Input: dimensioned drawing with shaded views. Units: mm. Origin: part minimum x, y, z. A direction names the side the tool comes from. Coordinates: 2 decimals unless noted, no trailing zeros. Order: outer loops, then holes, each group sorted by start corner. A loop starts at its lowest first (then second) coordinate and runs counter-clockwise, first axis right, second up. Notation, with made-up numbers: (69, 75) -> (124, 75) arc R19 cw to (124, 101) -> close; hole circle Ø10 at (60, 0). An arc over 180 degrees is marked (long way). Answer as CSV lines item,"result".
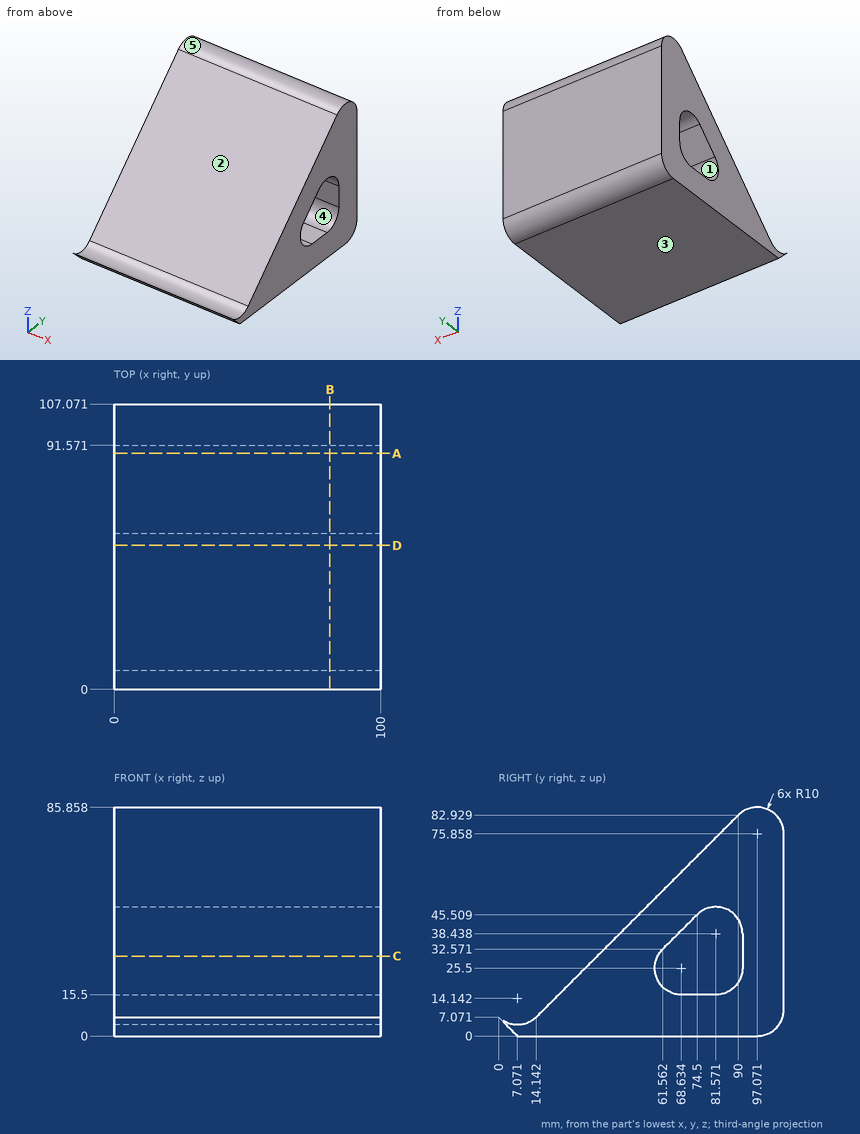
1. Contact query for flat-ended pins moving along their axis: pin 1 (14 mm diameter, centred on x = 53.5, y = 78, fed in from +Z); pin 2 (6.5 mm diameter, centred on x = 44.5, z = 29.5, fed in from -Y); pin 3 (12 mm diameter, centred on x = 54, y = 13.5, fed in from +Z). Output: stop coordinate, or through.
Findings:
pin 1,"stops at z = 77.93"
pin 2,"stops at y = 33.32"
pin 3,"stops at z = 12.43"
2. Cut plane D-D (y = 54). Return the cut outline in (x, z).
Findings:
outline,"(0, 0) -> (100, 0) -> (100, 46.93) -> (0, 46.93) -> close"
3. Mould query, pull axis Z, two halves, no side actions, for the marked faces 1, 2 and 3. Classes: released by +Z, released by -Z, zero draft, split by the parting line, or undercut.
Findings:
face 1,"undercut"
face 2,"released by +Z"
face 3,"released by -Z"
4. Cut plane C-C (z = 30). Return the cut outline in (x, y), plus the area to 3 significant figures.
Findings:
outline,"(0, 37.07) -> (100, 37.07) -> (100, 59.7) -> (0, 59.7) -> close; (0, 91.57) -> (100, 91.57) -> (100, 107.07) -> (0, 107.07) -> close"
area,"3,810 mm2"
5. Cut plane B-B (x = 81). Return the cut outline in (y, z), plus the area to 3 significant figures.
Findings:
outline,"(0, 7.07) -> (7.07, 0) -> (97.07, 0) arc R10 ccw to (107.07, 10) -> (107.07, 75.86) arc R10 ccw to (90, 82.93) -> (14.14, 7.07) arc R10 cw to start; hole (61.56, 32.57) arc R10 ccw to (68.63, 15.5) -> (81.57, 15.5) arc R10 ccw to (91.57, 25.5) -> (91.57, 38.44) arc R10 ccw to (74.5, 45.51) -> close"
area,"4,040 mm2"
6. Reachability of the marked faces 4 and 5 from +Z, -Z, +X, -X, +Y, -Y: full face, straight path, thin tool, end or side. Return the list, or none.
Findings:
face 4,"+X, -X"
face 5,"+Z, +X, -X"
7. Cut plane A-A (y = 88.5). Return the cut outline in (x, z).
Findings:
outline,"(0, 0) -> (100, 0) -> (100, 18.29) -> (0, 18.29) -> close; (0, 45.65) -> (100, 45.65) -> (100, 81.43) -> (0, 81.43) -> close"
8. Ray query, line 1 along Y through (x, z) = (45, 41) (1 decimal); line 2 along Y through (x, z) = (4.5, 41.5); line 3 along Z through (x, y) = (36, 74). Return the intervals inside material, ascending.
Findings:
line 1,"y = 48.1 to 70, 91.2 to 107.1"
line 2,"y = 48.57 to 70.49, 91.09 to 107.07"
line 3,"z = 0 to 15.5, 45.01 to 66.93"
